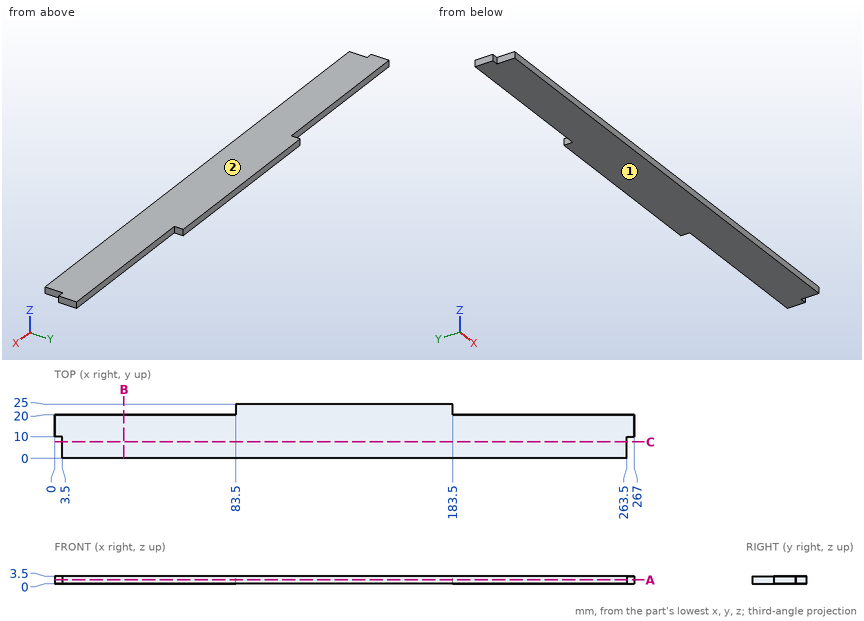
Design review of the part shown in the three views and the two pictorial views. Dimensions are in mm from the part's minimum x, y and z. Coordinates: 2 decimals unless noted, no trailing zeros. Order: outer loops, then holes, each group sorted by start corner. A loop starts at its lowest first (then second) coordinate and runs counter-clockwise, first axis right, second up.
Item 1: For line 1 (X direction, y = 20.5, z = 0.7); line 2 (Y direction, x = 34.5, z = 0.4); line 3 (X direction, y = 9, z = 1.5), list the stretches that pass through material, from the lowest coordinate up.
Item 2: Take a section at C-C, the plane y = 7.5. Write out the cut boundary in (x, z).
Item 3: The part is to be moulded in two halves that separate along Z. For the marked faces 1 and 2, say which applies: pulls with the +Z half, pulls with the -Z half, needs draft (parallel to the pull), parting line crosses it, or undercut.
Item 4: For pin 1 Ø5 at (x, y) = (224.5, 10.5) entering from -Z; pin 2 Ø1.8 at (x, z) = (220, 2) entering from +Y; pin 3 Ø1 at (x, z) = (265, 1) entering from -Y, all flat-tipped, find the tip position at first contact; note any pin that passes through.
Item 5: Take a section at B-B, the plane x = 32. Write out the cut boundary in (y, z).
Item 6: Take a section at A-A, the plane z = 1.9. Write out the cut boundary in (x, y).
The answers:
1. line 1: x = 83.5 to 183.5
1. line 2: y = 0 to 20
1. line 3: x = 3.5 to 263.5
2. outline: (3.5, 0) - (263.5, 0) - (263.5, 3.5) - (3.5, 3.5) - close
3. face 1: pulls with the -Z half
3. face 2: pulls with the +Z half
4. pin 1: stops at z = 0
4. pin 2: stops at y = 20
4. pin 3: stops at y = 10
5. outline: (0, 0) - (20, 0) - (20, 3.5) - (0, 3.5) - close
6. outline: (0, 10) - (3.5, 10) - (3.5, 0) - (263.5, 0) - (263.5, 10) - (267, 10) - (267, 20) - (183.5, 20) - (183.5, 25) - (83.5, 25) - (83.5, 20) - (0, 20) - close
